CAD build for the part. Positions are in the model's coordinates, mm. Round coordinates to 2 decimals unless told otherwise and drop trailing zeros. Write each loop counter-clockwise with the first axis right and the second up, starting at its lowest first coordinate (ties: lowest second). Pieces come first, ordered by that corner, then holes. Notation, with made-up numbers: (89.5, 8) - (144.5, 8) arc R29 cw to (144.5, 30) - close; hole circle Ø1 at (12.5, 50.25). An arc over 180 degrees is marked (long way). Use one line per item in the form item = value. Start each with the question number.
Item 1: Drill centre lines: L1, parallel to X at y = 478, z = 1.25; L2, parallel to Y at x = 434, z = 6.5; L3, parallel to X at y = -297.5, z = 8. Where is each one in solid material? Low to high.
Item 2: Band-saw the part on A-A, the plane z = 4.5. List the corners of the cut face in (x, y), and give its area (3 significant figures).
Item 3: Band-saw the part on B-B, the plane y = 559. List the corners of the cut face in (x, z), and give its area (3 significant figures).
Item 4: Band-saw the part on C-C, the plane x = -200. List the corners of the cut face in (y, z).
Item 5: Pin check, flat tips, straight feed: pin 1 (5 mm diameter, centred on y = 317.5, z = 7, fed in from -X); pin 2 (6.5 mm diameter, centred on y = 609.5, z = 5.5, fed in from +X); pin 3 (1.5 mm diameter, centred on x = 291, z = 7, fed in from -Y). Stop position of each tip, or through.
from build123d import *

# Parameters (mm, degrees)
F0_W     = 101.6
F0_H     = 581.585099
F1_DEPTH = 12.7


with BuildPart() as f1:
    # F0 (on Top) → F1 (new body)
    with BuildSketch(Plane.XY):
        with Locations((-236.551933, 473.884111)):
            Rectangle(F0_W, F0_H)
        Polygon((-185.751933, 183.091562), (-287.351933, 183.091562), (-300.051933, 183.091562), (-300.051933, 56.091562), (-218.208847, 56.091562), (410.263863, -418.272025), (505.818866, -363.103319), (-173.051933, 149.300135), (-173.051933, 183.091562), align=None)
        Polygon((513.583823, -358.620219), (505.818866, -363.103319), (410.263863, -418.272025), (403.598596, -422.120219), (467.098596, -532.105445), (577.083823, -468.605445), align=None)
    extrude(amount=F1_DEPTH)


solid = f1.part
Determined:
q1.L1 = -287.35 to -185.75
q1.L2 = -474.78 to -308.9
q1.L3 = 250.26 to 418.9
q2.outline = (-300.05, 56.09) - (-218.21, 56.09) - (410.26, -418.27) - (403.6, -422.12) - (467.1, -532.11) - (577.08, -468.61) - (513.58, -358.62) - (505.82, -363.1) - (-173.05, 149.3) - (-173.05, 183.09) - (-185.75, 183.09) - (-185.75, 764.68) - (-287.35, 764.68) - (-287.35, 183.09) - (-300.05, 183.09) - close
q2.area = 172,000 mm²
q3.outline = (-287.35, 0) - (-185.75, 0) - (-185.75, 12.7) - (-287.35, 12.7) - close
q3.area = 1,290 mm²
q4.outline = (42.35, 0) - (764.68, 0) - (764.68, 12.7) - (42.35, 12.7) - close
q5.pin_1 = -287.35
q5.pin_2 = -185.75
q5.pin_3 = -328.82
